from build123d import *

# Parameters (mm, degrees)
BASE_EXTRUDE_START               = -71
BASE_EXTRUDE_DEPTH               = 71
SKETCH2_R                        = 6
CUT_EXTRUDE1_DEPTH               = 69.7
SKETCH4_R                        = 6
BOSS_EXTRUDE1_DEPTH              = 10
CUT_EXTRUDE3_REACH               = 75.248
SKETCH19_R                       = 3
F_10_32_TAPPED_HOLE1_D           = 4.0386
F_10_32_TAPPED_HOLE1_DEPTH       = 13.6144
F_10_32_TAPPED_HOLE1_CBORE_D     = 4.826
F_10_32_TAPPED_HOLE1_CBORE_DEPTH = 9.652
F_10_32_TAPPED_HOLE1_TIP         = 1.213317848
F_4_40_TAPPED_HOLE1_D            = 2.2606
F_4_40_TAPPED_HOLE1_DEPTH        = 8.8646
F_4_40_TAPPED_HOLE1_CBORE_D      = 2.8448
F_4_40_TAPPED_HOLE1_CBORE_DEPTH  = 5.6896
F_4_40_TAPPED_HOLE1_TIP          = 0.679152758
HOLE1_D                          = 4
HOLE1_DEPTH                      = 3.5
CUT_EXTRUDE4_DEPTH               = 3.5
F_10_32_TAPPED_HOLE2_D           = 4.0386
F_10_32_TAPPED_HOLE2_DEPTH       = 13.6144
F_10_32_TAPPED_HOLE2_CBORE_D     = 4.826
F_10_32_TAPPED_HOLE2_CBORE_DEPTH = 9.652
F_10_32_TAPPED_HOLE2_TIP         = 1.213317848
SKETCH30_W                       = 28
SKETCH30_H                       = 31
BOSS_EXTRUDE2_DEPTH              = 8
BOSS_EXTRUDE3_DEPTH              = 3
SKETCH35_R                       = 2
BOSS_EXTRUDE5_DEPTH              = 3
CHAMFER2_SIZE                    = 0.5
BOSS_EXTRUDE6_DEPTH              = 8
BOSS_EXTRUDE7_DEPTH              = 3
CUT_EXTRUDE7_REACH               = 97.076
SKETCH38_R                       = 5
CUT_EXTRUDE8_REACH               = 112.864
SKETCH46_R                       = 5
CHAMFER3_SIZE                    = 0.5


with BuildPart() as part:
    # Sketch1 → Base-Extrude (new body)
    with BuildSketch(Plane(origin=(0, 0, 53.15), x_dir=(-1, 0, 0), z_dir=(0, 0, 1)).offset(BASE_EXTRUDE_START)):
        with BuildLine():
            Line((22.365, 8.6741), (23, 8.0391))
            Line((23, 8.0391), (23, -8.0391))
            Line((23, -8.0391), (22.365, -8.6741))
            Line((22.365, -8.6741), (8.135, -8.6741))
            Line((8.135, -8.6741), (7.5, -8.0391))
            Line((7.5, -8.0391), (-7.5, -8.0391))
            Line((-7.5, -8.0391), (-8.135, -8.6741))
            Line((-8.135, -8.6741), (-22.365, -8.6741))
            Line((-22.365, -8.6741), (-23, -8.0391))
            Line((-23, -8.0391), (-23, -4.5593))
            Line((-23, -4.5593), (-21.70268423, -4.5593))
            ThreePointArc((-21.70268423, -4.5593), (-18.120014782, -3.0226), (-21.70268423, -1.4859))
            Line((-21.70268423, -1.4859), (-23, -1.4859))
            Line((-23, -1.4859), (-23, 1.4859))
            Line((-23, 1.4859), (-21.70268423, 1.4859))
            ThreePointArc((-21.70268423, 1.4859), (-18.120014782, 3.0226), (-21.70268423, 4.5593))
            Line((-21.70268423, 4.5593), (-23, 4.5593))
            Line((-23, 4.5593), (-23, 8.0391))
            Line((-23, 8.0391), (-22.365, 8.6741))
            Line((-22.365, 8.6741), (-8.135, 8.6741))
            Line((-8.135, 8.6741), (-7.5, 8.0391))
            Line((-7.5, 8.0391), (7.5, 8.0391))
            Line((7.5, 8.0391), (8.135, 8.6741))
            Line((8.135, 8.6741), (22.365, 8.6741))
        make_face()
    extrude(amount=BASE_EXTRUDE_DEPTH)

    # Sketch2 → Cut-Extrude1 (cut)
    with BuildSketch(Plane(origin=(0, 0, 53.15), x_dir=(-1, 0, 0), z_dir=(0, 0, -1))):
        with Locations(Location((-11.0744, 0, 0), (0, 0, 180))):
            Circle(SKETCH2_R)
        with Locations(Location((10.5156, 0, 0), (0, 0, 180))):
            Circle(SKETCH2_R)
    extrude(amount=CUT_EXTRUDE1_DEPTH, mode=Mode.SUBTRACT)

    # Sketch4 → Boss-Extrude1 (add)
    with BuildSketch(Plane.XY.offset(51.15)):
        with Locations((11.0744, 0)):
            Circle(SKETCH4_R)
        with Locations((-10.5156, 0)):
            Circle(SKETCH4_R)
    extrude(amount=-BOSS_EXTRUDE1_DEPTH)

    # Sketch19 → Cut-Extrude3 (cut, up to next)
    with BuildSketch(Plane.XY.offset(51.15), mode=Mode.PRIVATE) as cut_extrude3_sk1:
        with Locations((11.0744, 0)):
            Circle(SKETCH19_R)
    cut_extrude3_tool1 = extrude(cut_extrude3_sk1.sketch, amount=-CUT_EXTRUDE3_REACH, mode=Mode.PRIVATE) & part.part
    # Sketch19 → Cut-Extrude3 (cut, up to next)
    with BuildSketch(Plane.XY.offset(51.15), mode=Mode.PRIVATE) as cut_extrude3_sk2:
        with Locations((-10.5156, 0)):
            Circle(SKETCH19_R)
    cut_extrude3_tool2 = extrude(cut_extrude3_sk2.sketch, amount=-CUT_EXTRUDE3_REACH, mode=Mode.PRIVATE) & part.part
    add(cut_extrude3_tool1.solids().sort_by_distance((11.0744, 0, 51.15))[0], mode=Mode.SUBTRACT)
    add(cut_extrude3_tool2.solids().sort_by_distance((-10.5156, 0, 51.15))[0], mode=Mode.SUBTRACT)

    # #10-32 Tapped Hole1
    with Locations(Plane.XZ.offset(8.0391)):
        with Locations((0, 30.15), (0, 0.15)):
            CounterBoreHole(F_10_32_TAPPED_HOLE1_D / 2, F_10_32_TAPPED_HOLE1_CBORE_D / 2, F_10_32_TAPPED_HOLE1_CBORE_DEPTH, depth=F_10_32_TAPPED_HOLE1_DEPTH)
            with Locations((0, 0, -(F_10_32_TAPPED_HOLE1_DEPTH + F_10_32_TAPPED_HOLE1_TIP / 2))):  # 118° drill point
                Cone(0, F_10_32_TAPPED_HOLE1_D / 2, F_10_32_TAPPED_HOLE1_TIP, mode=Mode.SUBTRACT)

    # #4-40 Tapped Hole1
    with Locations(Plane(origin=(0, 0, -17.85), x_dir=(-1, 0, 0), z_dir=(0, 0, -1))):
        with Locations((20, -4.6741), (20, 4.3259), (-3, -4.6741), (-3, 4.3259)):
            CounterBoreHole(F_4_40_TAPPED_HOLE1_D / 2, F_4_40_TAPPED_HOLE1_CBORE_D / 2, F_4_40_TAPPED_HOLE1_CBORE_DEPTH, depth=F_4_40_TAPPED_HOLE1_DEPTH)
            with Locations((0, 0, -(F_4_40_TAPPED_HOLE1_DEPTH + F_4_40_TAPPED_HOLE1_TIP / 2))):  # 118° drill point
                Cone(0, F_4_40_TAPPED_HOLE1_D / 2, F_4_40_TAPPED_HOLE1_TIP, mode=Mode.SUBTRACT)

    # Hole1
    with Locations(Plane.XZ.offset(8.6741)):
        with Locations((-19, 39.65)):
            Hole(HOLE1_D / 2, depth=HOLE1_DEPTH)

    # Sketch27 → Cut-Extrude4 (cut)
    with BuildSketch(Plane.XZ.offset(8.6741)):
        with BuildLine():
            Line((-21, 5.15), (-21, 4.15))
            ThreePointArc((-21, 4.15), (-19, 2.15), (-17, 4.15))
            Line((-17, 4.15), (-17, 5.15))
            ThreePointArc((-17, 5.15), (-19, 7.15), (-21, 5.15))
        make_face()
    extrude(amount=-CUT_EXTRUDE4_DEPTH, mode=Mode.SUBTRACT)

    # #10-32 Tapped Hole2
    with Locations(Plane.ZY.offset(23)):
        with Locations((34.55, -0.1741), (-14.05, -0.1741)):
            CounterBoreHole(F_10_32_TAPPED_HOLE2_D / 2, F_10_32_TAPPED_HOLE2_CBORE_D / 2, F_10_32_TAPPED_HOLE2_CBORE_DEPTH, depth=F_10_32_TAPPED_HOLE2_DEPTH)
            with Locations((0, 0, -(F_10_32_TAPPED_HOLE2_DEPTH + F_10_32_TAPPED_HOLE2_TIP / 2))):  # 118° drill point
                Cone(0, F_10_32_TAPPED_HOLE2_D / 2, F_10_32_TAPPED_HOLE2_TIP, mode=Mode.SUBTRACT)

    # Sketch30 → Boss-Extrude2 (add)
    with BuildSketch(Plane(origin=(0, 0, -17.85), x_dir=(-1, 0, 0), z_dir=(0, 0, -1))):
        with Locations((8.5, 7.9609)):
            Rectangle(SKETCH30_W, SKETCH30_H)
    extrude(amount=BOSS_EXTRUDE2_DEPTH)

    # Sketch31 → Boss-Extrude3 (add)
    with BuildSketch(Plane(origin=(0, 0, -25.85), x_dir=(-1, 0, 0), z_dir=(0, 0, -1))):
        Polygon((19.42820323, 16.4609), (15.964101615, 22.4609), (9.035898385, 22.4609), (5.57179677, 16.4609), (9.035898385, 10.4609), (15.964101615, 10.4609), align=None)
    extrude(amount=BOSS_EXTRUDE3_DEPTH)

    # Sketch35 → Boss-Extrude5 (add)
    with BuildSketch(Plane(origin=(0, 0, -25.85), x_dir=(-1, 0, 0), z_dir=(0, 0, -1))):
        with Locations((20, 4.3259)):
            Circle(SKETCH35_R)
        with Locations((-3, 4.3259)):
            Circle(SKETCH35_R)
        with Locations((-3, -4.6741)):
            Circle(SKETCH35_R)
        with Locations((20, -4.6741)):
            Circle(SKETCH35_R)
    extrude(amount=BOSS_EXTRUDE5_DEPTH)

    # Chamfer2
    chamfer2_edges = [part.edges().sort_by_distance(p)[0] for p in [
        (-18, 4.3259, -28.85),
        (5, 4.3259, -28.85),
        (5, -4.6741, -28.85),
        (-18, -4.6741, -28.85),
    ]]
    chamfer(chamfer2_edges, length=CHAMFER2_SIZE)

    # Sketch36 → Boss-Extrude6 (add)
    with BuildSketch(Plane.XY.offset(43.15)):
        Polygon((-23.5, 23.3259), (-23.5, 6.6741), (-23, 6.6741), (-23, -6.6741), (-40, -6.6741), (-40, 23.3259), align=None)
    extrude(amount=BOSS_EXTRUDE6_DEPTH)

    # Sketch37 → Boss-Extrude7 (add)
    with BuildSketch(Plane.XY.offset(51.15)):
        Polygon((-28.535898385, 22.8259), (-35.464101615, 22.8259), (-38.92820323, 16.8259), (-35.464101615, 10.8259), (-28.535898385, 10.8259), (-25.07179677, 16.8259), align=None)
    extrude(amount=BOSS_EXTRUDE7_DEPTH)

    # Sketch38 → Cut-Extrude7 (cut, up to next)
    with BuildSketch(Plane.XY.offset(54.15), mode=Mode.PRIVATE) as cut_extrude7_sk1:
        with Locations((-32, 16.8259)):
            Circle(SKETCH38_R)
    cut_extrude7_tool1 = extrude(cut_extrude7_sk1.sketch, amount=-CUT_EXTRUDE7_REACH, mode=Mode.PRIVATE) & part.part
    add(cut_extrude7_tool1.solids().sort_by_distance((-32, 16.8259, 54.15))[0], mode=Mode.SUBTRACT)

    # Sketch44 → Boss-Revolve1 (revolve)
    with BuildSketch(Plane(origin=(0, 16.8259, 0), x_dir=(-1, 0, 0), z_dir=(0, 1, 0)), mode=Mode.PRIVATE) as boss_revolve1_sk:
        Polygon((32, 71.85), (37, 71.85), (37, 43.65), (36.5, 43.15), (32, 43.15), align=None)
    revolve(boss_revolve1_sk.sketch.rotate(Axis((-32, 16.8259, 54.15), (0, 0, -1)), 180), axis=Axis((-32, 16.8259, 54.15), (0, 0, -1)))

    # Sketch46 → Cut-Extrude8 (cut, up to next)
    with BuildSketch(Plane(origin=(0, 0, -28.85), x_dir=(-1, 0, 0), z_dir=(0, 0, -1)), mode=Mode.PRIVATE) as cut_extrude8_sk1:
        with Locations((12.5, 16.4609)):
            Circle(SKETCH46_R)
    cut_extrude8_tool1 = extrude(cut_extrude8_sk1.sketch, amount=-CUT_EXTRUDE8_REACH, mode=Mode.PRIVATE) & part.part
    add(cut_extrude8_tool1.solids().sort_by_distance((-12.5, 16.4609, -28.85))[0], mode=Mode.SUBTRACT)

    # Sketch47 → Boss-Revolve2 (revolve)
    with BuildSketch(Plane(origin=(0, 16.4609, 0), x_dir=(-1, 0, 0), z_dir=(0, 1, 0))):
        Polygon((17, -17.85), (12.5, -17.85), (12.5, -46.55), (17.5, -46.55), (17.5, -18.35), align=None)
    revolve(axis=Axis((-12.5, 16.4609, -17.85), (0, 0, -1)))

    # Chamfer3
    chamfer3_edges = [part.edges().sort_by_distance(p)[0] for p in [
        (-37, 16.8259, 71.85),
        (-7.5, 16.4609, -46.55),
    ]]
    chamfer(chamfer3_edges, length=CHAMFER3_SIZE)


solid = part.part
Input: part model. Units: mm. Frame: model coordinates. A direction names the side the tool comes from. Give positions to 0.01 mm unless a question says otherwise; leave off trailing zeros. Order: outer loops, then holes, each group sorted by start corner. A loop starts at its lowest first (then second) coordinate and runs counter-clockwise, first axis right, second up. Notation, with made-up numbers: (34, -6.75) - (79, -6.75) arc R25 cw to (79, 6.25) - close; hole circle Ø1 at (-27.5, 16). An arc over 180 degrees is marked (long way). Answer as a JSON object with one key per item and string values. Group by question number.
Q1. First-contact query: pin 1 Ø2 at (x, y) = (2, 6.5) entering from -Z; pin 2 Ø3.5 at (x, y) = (-20, -4.67) entering from +Z; pin 3 Ø3 at (x, z) = (10.5, 49.5) entering from +Y; pin 4 Ø4 at (y, z) = (12, -10) entering from -X. Flat tips, straight axial feed; report the tip coordinate or a pass-through.
Q2. Cut plane B-B, the plane x = -32. Output: boundary loops of the cut face in (y, z), then the cut area to 4 significant figures.
Q3. Cut plane A-A, the plane z = 39.65. Count the separate pieces of the cut face and the enclosed holes in it, then the cut area to 3 significant figures.
Q4. Mould query, pull axis Y, two halves, no side actions, for faces 5 (the face through (-32, 23.326, 47)), 6 (the face through (-32, 17, 71.85)), 7 (the face through (-20, -5, -17.85)). Classes: pulls with the +Y half, pulls with the -Y half, needs draft (parallel to the pull), parting line crosses it, or undercut.
Q5. Line query: probe 1 along Z at (x, y) = (15, -1.5); probe 2 along Y at (x, z) = (-18.5, -14.05); probe 3 along X at (y, z) = (2.5, 1). Output: solid intervals per line, ascending.
Q6. Cut plane C-C, the plane z = 16. Output: boundary loops of the cut face in (x, y) (3 decimals).
Q7. Cut plane D-D, the plane z = -30. Output: boundary loops of the cut face in (x, y), then the cut area to 3 significant figures.
Q8. Set-up query: faces 1 (the face through (-9, 3, 51.15)), 2 (the face through (-18.956, 3.893, -10.551)), 3 (the face through (0.263, 3.622, 32.152)), 4 (the face through (-13, 22.461, -27)). Return all of +Z, -Z, +X, -X, +Y, -Y with unobstructed straight access to the full face (end or side cutting, diameter ignored); none if empty.
Results:
{
 "1": {"pin 1": "z = -28.85", "pin 2": "z = 53.15", "pin 3": "y = 8.67", "pin 4": "through"},
 "2": {"outline": "(-6.67, 43.15) - (11.83, 43.15) - (11.83, 43.65) - (12.33, 43.15) - (21.33, 43.15) - (21.83, 43.65) - (21.83, 43.15) - (23.33, 43.15) - (23.33, 51.15) - (22.83, 51.15) - (22.83, 54.15) - (21.83, 54.15) - (21.83, 71.35) - (21.33, 71.85) - (12.33, 71.85) - (11.83, 71.35) - (11.83, 54.15) - (10.83, 54.15) - (10.83, 51.15) - (-6.67, 51.15) - close", "area": "452.5 mm^2"},
 "3": {"separate pieces": "1", "enclosed holes": "2", "area": "504 mm^2"},
 "4": {"face 5": "pulls with the +Y half", "face 6": "needs draft", "face 7": "undercut"},
 "5": {"probe 1": "-17.85 to -16.55, 41.15 to 51.15", "probe 2": "-8.67 to -2.59, 2.24 to 8.67", "probe 3": "-23 to -15.97, -5.06 to -1.83, 1.83 to 5.62, 16.53 to 18.19"},
 "6": {"outline": "(-23, -8.039) - (-22.365, -8.674) - (-8.135, -8.674) - (-7.5, -8.039) - (7.5, -8.039) - (8.135, -8.674) - (22.365, -8.674) - (23, -8.039) - (23, -4.559) - (21.703, -4.559) arc R2.121 cw (long way) to (21.703, -1.486) - (23, -1.486) - (23, 1.486) - (21.703, 1.486) arc R2.121 cw (long way) to (21.703, 4.559) - (23, 4.559) - (23, 8.039) - (22.365, 8.674) - (8.135, 8.674) - (7.5, 8.039) - (-7.5, 8.039) - (-8.135, 8.674) - (-22.365, 8.674) - (-23, 8.039) - close; hole circle Ø12 at (-10.516, 0); hole circle Ø12 at (11.074, 0)"},
 "7": {"outline": "circle Ø10 at (-12.5, 16.46)", "area": "78.5 mm^2"},
 "8": {"face 1": "+Z", "face 2": "none", "face 3": "-Y", "face 4": "-Z, +X, -X, +Y"}
}
